Source: CAD feature listing. Evaluate the final solid. Frame: model axes, mm. A direction names the side the tool comes from. Give positions to 0.01 mm unless a question says otherwise; leave off trailing zeros. Loops run counter-clockwise (first coordinate to the right, second up) from the corner with the lowest first, then second, coordinate; pieces in that order, holes last. Notation, with made-up numbers: M -19,4.25 L -1,4.25 A24 cw -1,23.25 Z; hole C -17.5,21.5 d9. An arc over 180 degrees is marked long. Answer in a Markdown table with one row per item.
```python
from build123d import *

# Parameters (mm, degrees)
BOSS_EXTRUDE1_DEPTH                             = 1.5
SKETCH2_R                                       = 2.5
CUT_EXTRUDE1_DEPTH                              = 2.5
CUT_EXTRUDE1_DEPTH_BACK                         = 2.5
SKETCH4_W                                       = 18.7
SKETCH4_H                                       = 38.8
CUT_EXTRUDE4_DEPTH                              = 2.5
SKETCH4_2_W                                     = 18.7
SKETCH4_2_H                                     = 38.8
CUT_EXTRUDE5_DEPTH                              = 0.3
FILLET6_R                                       = 2
SKETCH4_4_W                                     = 18.7
SKETCH4_4_H                                     = 38.8
CUT_EXTRUDE6_DEPTH                              = 0.5
CUT_EXTRUDE6_DEPTH_BACK                         = 0.3
BOSS_EXTRUDE2_DEPTH                             = 0.8
FILLET7_R                                       = 2
CHAMFER1_SIZE                                   = 3
FILLET2_R                                       = 1
FILLET3_R                                       = 3
CUT_EXTRUDE7_DEPTH                              = 0.75
CSK_FOR_M2_FLAT_HEAD_MACHINE_SCREW1_D           = 2.4
CSK_FOR_M2_FLAT_HEAD_MACHINE_SCREW1_DEPTH       = 4
CSK_FOR_M2_FLAT_HEAD_MACHINE_SCREW1_CSINK_D     = 4.4
CSK_FOR_M2_FLAT_HEAD_MACHINE_SCREW1_CSINK_ANGLE = 90
CSK_FOR_M2_FLAT_HEAD_MACHINE_SCREW1_TIP         = 0.721032743


with BuildPart() as part:
    # Sketch1 → Boss-Extrude1 (new body, symmetric)
    with BuildSketch(Plane(origin=(0, 0, 0), x_dir=(1, 0, 0), z_dir=(0, 1, 0))):
        Polygon((-9, 0), (-9, 10), (-7.5, 10.779220779), (-7.5, 13.779220779), (-11.35, 15.779220779), (-11.35, 35.779220779), (6.35, 55.779220779), (11.35, 55.779220779), (11.35, 15.779220779), (7.5, 13.779220779), (7.5, 10.779220779), (9, 10), (9, 0), align=None)
    extrude(amount=BOSS_EXTRUDE1_DEPTH, both=True)

    # Sketch2 → Cut-Extrude1 (cut, two sides)
    with BuildSketch(Plane(origin=(0, 0, 0), x_dir=(1, 0, 0), z_dir=(0, 1, 0))) as cut_extrude1_sk:
        with Locations((-5, 5)):
            Circle(SKETCH2_R)
        with Locations((5, 5)):
            Circle(SKETCH2_R)
    extrude(amount=CUT_EXTRUDE1_DEPTH, mode=Mode.SUBTRACT)
    extrude(cut_extrude1_sk.sketch, amount=-CUT_EXTRUDE1_DEPTH_BACK, mode=Mode.SUBTRACT)

    # Sketch4 → Cut-Extrude4 (cut, through all)
    with BuildSketch(Plane(origin=(0, 0, 0), x_dir=(1, 0, 0), z_dir=(0, 1, 0))):
        with Locations((0, 36.379220779)):
            Rectangle(SKETCH4_W, SKETCH4_H)
    extrude(amount=CUT_EXTRUDE4_DEPTH, mode=Mode.SUBTRACT)

    # Sketch4<2> → Cut-Extrude5 (cut, symmetric)
    with BuildSketch(Plane(origin=(0, 0, 0), x_dir=(1, 0, 0), z_dir=(0, 1, 0))):
        with Locations((0, 36.379220779)):
            Rectangle(SKETCH4_2_W, SKETCH4_2_H)
    extrude(amount=CUT_EXTRUDE5_DEPTH, both=True, mode=Mode.SUBTRACT)

    # Fillet6
    fillet6_edges = [part.edges().sort_by_distance(p)[0] for p in [
        (-9.35, 0.6, -16.979220779),
    ]]
    fillet(fillet6_edges, radius=FILLET6_R)

    # Sketch4<4> → Cut-Extrude6 (cut, two sides)
    with BuildSketch(Plane(origin=(0, 0, 0), x_dir=(1, 0, 0), z_dir=(0, 1, 0))) as cut_extrude6_sk:
        with Locations((0, 36.379220779)):
            Rectangle(SKETCH4_4_W, SKETCH4_4_H)
    extrude(amount=CUT_EXTRUDE6_DEPTH, mode=Mode.SUBTRACT)
    extrude(cut_extrude6_sk.sketch, amount=-CUT_EXTRUDE6_DEPTH_BACK, mode=Mode.SUBTRACT)

    # Sketch9 → Boss-Extrude2 (add)
    with BuildSketch(Plane(origin=(0, -0.3, 0), x_dir=(1, 0, 0), z_dir=(0, 1, 0))):
        Polygon((9.35, 16.979220779), (9.35, 31.104220779), (-7.35, 18.489915966), (-9.35, 16.979220779), align=None)
    extrude(amount=BOSS_EXTRUDE2_DEPTH)

    # Fillet7
    fillet7_edges = [part.edges().sort_by_distance(p)[0] for p in [
        (9.35, 1, -16.979220779),
    ]]
    fillet(fillet7_edges, radius=FILLET7_R)

    # Chamfer1
    chamfer1_edges = [part.edges().sort_by_distance(p)[0] for p in [
        (-9, 0, 0),
        (9, 0, 0),
    ]]
    chamfer(chamfer1_edges, length=CHAMFER1_SIZE)

    # Fillet2
    fillet2_edges = [part.edges().sort_by_distance(p)[0] for p in [
        (-9, 0, -10),
        (-7.5, 0, -10.779220779),
        (-7.5, 0, -13.779220779),
        (-11.35, 0, -15.779220779),
        (11.35, 0, -15.779220779),
        (7.5, 0, -13.779220779),
        (7.5, 0, -10.779220779),
        (9, 0, -10),
    ]]
    fillet(fillet2_edges, radius=FILLET2_R)

    # Fillet3
    fillet3_edges = [part.edges().sort_by_distance(p)[0] for p in [
        (9, 0, -3),
        (-6, 0, 0),
        (6, 0, 0),
        (-9, 0, -3),
    ]]
    fillet(fillet3_edges, radius=FILLET3_R)

    # Sketch10 → Cut-Extrude7 (cut)
    with BuildSketch(Plane(origin=(0, 1.5, 0), x_dir=(1, 0, 0), z_dir=(0, 1, 0))):
        with BuildLine():
            Line((-10.35, 36.909164283), (-10.35, 18.97922078))
            ThreePointArc((-10.35, 18.97922078), (-10.152517077, 17.908754511), (-9.586067977, 16.97922078))
            Line((-9.586067977, 16.97922078), (9.586067977, 16.97922078))
            ThreePointArc((9.586067977, 16.97922078), (10.152517077, 17.908754511), (10.35, 18.97922078))
            Line((10.35, 18.97922078), (10.35, 55.77922078))
            Line((10.35, 55.77922078), (6.35, 55.77922078))
            Line((6.35, 55.77922078), (-10.35, 36.909164283))
        make_face()
    extrude(amount=-CUT_EXTRUDE7_DEPTH, mode=Mode.SUBTRACT)

    # CSK for M2 Flat Head Machine Screw1
    with Locations(Plane(origin=(-5, 1.5, 32.5), x_dir=(1, 0, 0), z_dir=(0, 1, 0))):
        with Locations((11.85, 56.367589763), (6.85, 52.590851795)):
            CounterSinkHole(CSK_FOR_M2_FLAT_HEAD_MACHINE_SCREW1_D / 2, CSK_FOR_M2_FLAT_HEAD_MACHINE_SCREW1_CSINK_D / 2, depth=CSK_FOR_M2_FLAT_HEAD_MACHINE_SCREW1_DEPTH, counter_sink_angle=CSK_FOR_M2_FLAT_HEAD_MACHINE_SCREW1_CSINK_ANGLE)
            with Locations((0, 0, -(CSK_FOR_M2_FLAT_HEAD_MACHINE_SCREW1_DEPTH + CSK_FOR_M2_FLAT_HEAD_MACHINE_SCREW1_TIP / 2))):  # 118° drill point
                Cone(0, CSK_FOR_M2_FLAT_HEAD_MACHINE_SCREW1_D / 2, CSK_FOR_M2_FLAT_HEAD_MACHINE_SCREW1_TIP, mode=Mode.SUBTRACT)


solid = part.part
```
1) Pin query (flat end, axial travel): pin 1 Ø4 at (x, z) = (1.85, -20.09) entering from +Y; pin 2 Ø0.5 at (y, z) = (0, -12.5) entering from +X; pin 3 Ø8 at (x, z) = (-2.5, -27.5) entering from +Y. Return the tip coordinate at first contact, or that it passes through.
Reply:
| item | result |
|---|---|
| pin 1 | stops at y = 0.5 |
| pin 2 | stops at x = 7.5 |
| pin 3 | stops at y = -0.3 |
2) Set-up query: faces 4 (the flat face through (-9.41, 0.02, -14.77)), 5 (the flat face through (10, 0.75, -35)), 6 (the flat face through (9, 0, -7)), 7 (the flat face through (0, 0, 0)), 8 (the cylindrical face through (-2.615, 0.021, -5.751)). Return all of +Z, -Z, +X, -X, +Y, -Y with unobstructed straight access to the full face (end or side cutting, diameter ignored); none if empty.
Reply:
| item | result |
|---|---|
| face 4 | -X, +Y, -Y |
| face 5 | -Z, +Y |
| face 6 | +Z, +X, +Y, -Y |
| face 7 | +Z, +X, -X, +Y, -Y |
| face 8 | +Y, -Y |
3) Section D-D, the plane z = -40.5. Return loops of the section in (x, y).
Reply:
| item | result |
|---|---|
| outline | M -7.17,-1.5 L 11.35,-1.5 L 11.35,1.5 L 10.35,1.5 L 10.35,0.75 L 9.35,0.75 L 9.35,-0.3 L -7.17,-0.3 Z |
4) Pull-direction query (X, two-part tool) for faces 1 (the flat face through (9.444, 0.021, -14.789)), 2 (the flat face through (0, 1, -16.979)), 3 (the flat face through (-2.624, -0.646, -45.639)); classes: released by +X, released by -X, zero draft, split by the parting line, or undercut.
Reply:
| item | result |
|---|---|
| face 1 | released by +X |
| face 2 | undercut |
| face 3 | released by -X |
5) Section B-B, the plane z = -24.5. Return loops of the section in (x, y).
Reply:
| item | result |
|---|---|
| outline | M -11.35,-1.5 L 5.83,-1.5 L 5.83,0.5 L 0.61,0.5 L 0.61,-0.3 L -9.35,-0.3 L -9.35,0.75 L -10.35,0.75 L -10.35,1.5 L -11.35,1.5 Z; M 7.87,-1.5 L 11.35,-1.5 L 11.35,1.5 L 10.35,1.5 L 10.35,0.75 L 9.35,0.75 L 9.35,0.5 L 7.87,0.5 Z |
6) Section A-A, the plane z = -5. Return loops of the section in (x, y).
Reply:
| item | result |
|---|---|
| outline | M -9,-1.5 L -7.5,-1.5 L -7.5,1.5 L -9,1.5 Z; M -2.5,-1.5 L 2.5,-1.5 L 2.5,1.5 L -2.5,1.5 Z; M 7.5,-1.5 L 9,-1.5 L 9,1.5 L 7.5,1.5 Z |
7) Material intervals for L1, parallel to X at y = 0.35, z = -5; L2, parallel to X at y = -1.35, z = -4.5; L3, parallel to Z at x = 6.85, y = -0.65, sorted ascending.
Reply:
| item | result |
|---|---|
| L1 | x = -9 to -7.5, -2.5 to 2.5, 7.5 to 9 |
| L2 | x = -9 to -7.45, -2.55 to 2.55, 7.45 to 9 |
| L3 | z = -55.78 to -25.07, -22.67 to -6.68, -3.32 to -0.85 |
8) Section C-C, the plane x = 1.85. Return loops of the section in (y, z).
Reply:
| item | result |
|---|---|
| outline | M -1.5,-50.69 L -0.3,-50.69 L -0.3,-25.44 L 0.5,-25.44 L 0.5,-21.29 L -1.5,-21.29 Z; M -1.5,-18.89 L 0.5,-18.89 L 0.5,-16.98 L 1.5,-16.98 L 1.5,0 L -1.5,0 Z |
